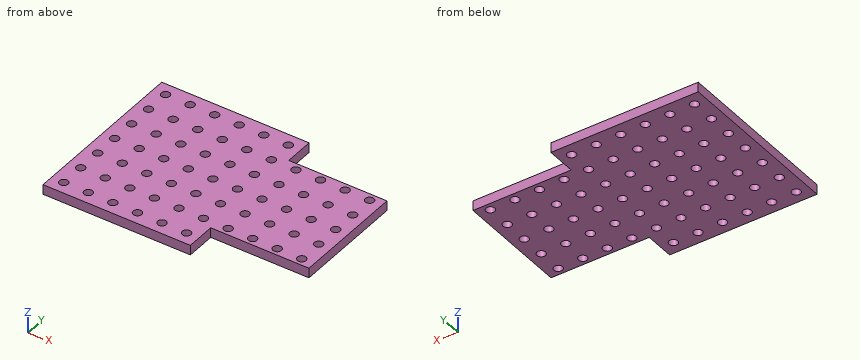
from build123d import *

# Parameters (mm, degrees)
ESQUISSE1_R        = 1.75
BOSS_EXTRU_1_DEPTH = 4


with BuildPart() as part:
    # Esquisse1 → Boss.-Extru.1 (new body)
    with BuildSketch(Plane.XY):
        Polygon((0, 0), (0, 70), (60, 70), (60, 58), (100, 58), (100, 12), (60, 12), (60, 0), align=None)
        with Locations((5, 5)):
            Circle(ESQUISSE1_R, mode=Mode.SUBTRACT)
        with Locations((15, 5)):
            Circle(ESQUISSE1_R, mode=Mode.SUBTRACT)
        with Locations((25, 5)):
            Circle(ESQUISSE1_R, mode=Mode.SUBTRACT)
        with Locations((35, 5)):
            Circle(ESQUISSE1_R, mode=Mode.SUBTRACT)
        with Locations((45, 5)):
            Circle(ESQUISSE1_R, mode=Mode.SUBTRACT)
        with Locations((55, 5)):
            Circle(ESQUISSE1_R, mode=Mode.SUBTRACT)
        with Locations((15, 15)):
            Circle(ESQUISSE1_R, mode=Mode.SUBTRACT)
        with Locations((25, 15)):
            Circle(ESQUISSE1_R, mode=Mode.SUBTRACT)
        with Locations((35, 15)):
            Circle(ESQUISSE1_R, mode=Mode.SUBTRACT)
        with Locations((45, 15)):
            Circle(ESQUISSE1_R, mode=Mode.SUBTRACT)
        with Locations((55, 15)):
            Circle(ESQUISSE1_R, mode=Mode.SUBTRACT)
        with Locations((65, 15)):
            Circle(ESQUISSE1_R, mode=Mode.SUBTRACT)
        with Locations((75, 15)):
            Circle(ESQUISSE1_R, mode=Mode.SUBTRACT)
        with Locations((85, 15)):
            Circle(ESQUISSE1_R, mode=Mode.SUBTRACT)
        with Locations((95, 15)):
            Circle(ESQUISSE1_R, mode=Mode.SUBTRACT)
        with Locations((15, 25)):
            Circle(ESQUISSE1_R, mode=Mode.SUBTRACT)
        with Locations((25, 25)):
            Circle(ESQUISSE1_R, mode=Mode.SUBTRACT)
        with Locations((35, 25)):
            Circle(ESQUISSE1_R, mode=Mode.SUBTRACT)
        with Locations((45, 25)):
            Circle(ESQUISSE1_R, mode=Mode.SUBTRACT)
        with Locations((55, 25)):
            Circle(ESQUISSE1_R, mode=Mode.SUBTRACT)
        with Locations((65, 25)):
            Circle(ESQUISSE1_R, mode=Mode.SUBTRACT)
        with Locations((75, 25)):
            Circle(ESQUISSE1_R, mode=Mode.SUBTRACT)
        with Locations((85, 25)):
            Circle(ESQUISSE1_R, mode=Mode.SUBTRACT)
        with Locations((95, 25)):
            Circle(ESQUISSE1_R, mode=Mode.SUBTRACT)
        with Locations((15, 35)):
            Circle(ESQUISSE1_R, mode=Mode.SUBTRACT)
        with Locations((25, 35)):
            Circle(ESQUISSE1_R, mode=Mode.SUBTRACT)
        with Locations((35, 35)):
            Circle(ESQUISSE1_R, mode=Mode.SUBTRACT)
        with Locations((45, 35)):
            Circle(ESQUISSE1_R, mode=Mode.SUBTRACT)
        with Locations((55, 35)):
            Circle(ESQUISSE1_R, mode=Mode.SUBTRACT)
        with Locations((65, 35)):
            Circle(ESQUISSE1_R, mode=Mode.SUBTRACT)
        with Locations((75, 35)):
            Circle(ESQUISSE1_R, mode=Mode.SUBTRACT)
        with Locations((85, 35)):
            Circle(ESQUISSE1_R, mode=Mode.SUBTRACT)
        with Locations((95, 35)):
            Circle(ESQUISSE1_R, mode=Mode.SUBTRACT)
        with Locations((15, 45)):
            Circle(ESQUISSE1_R, mode=Mode.SUBTRACT)
        with Locations((25, 45)):
            Circle(ESQUISSE1_R, mode=Mode.SUBTRACT)
        with Locations((35, 45)):
            Circle(ESQUISSE1_R, mode=Mode.SUBTRACT)
        with Locations((45, 45)):
            Circle(ESQUISSE1_R, mode=Mode.SUBTRACT)
        with Locations((55, 45)):
            Circle(ESQUISSE1_R, mode=Mode.SUBTRACT)
        with Locations((65, 45)):
            Circle(ESQUISSE1_R, mode=Mode.SUBTRACT)
        with Locations((75, 45)):
            Circle(ESQUISSE1_R, mode=Mode.SUBTRACT)
        with Locations((85, 45)):
            Circle(ESQUISSE1_R, mode=Mode.SUBTRACT)
        with Locations((95, 45)):
            Circle(ESQUISSE1_R, mode=Mode.SUBTRACT)
        with Locations((15, 55)):
            Circle(ESQUISSE1_R, mode=Mode.SUBTRACT)
        with Locations((25, 55)):
            Circle(ESQUISSE1_R, mode=Mode.SUBTRACT)
        with Locations((35, 55)):
            Circle(ESQUISSE1_R, mode=Mode.SUBTRACT)
        with Locations((45, 55)):
            Circle(ESQUISSE1_R, mode=Mode.SUBTRACT)
        with Locations((55, 55)):
            Circle(ESQUISSE1_R, mode=Mode.SUBTRACT)
        with Locations((65, 55)):
            Circle(ESQUISSE1_R, mode=Mode.SUBTRACT)
        with Locations((75, 55)):
            Circle(ESQUISSE1_R, mode=Mode.SUBTRACT)
        with Locations((85, 55)):
            Circle(ESQUISSE1_R, mode=Mode.SUBTRACT)
        with Locations((95, 55)):
            Circle(ESQUISSE1_R, mode=Mode.SUBTRACT)
        with Locations((15, 65)):
            Circle(ESQUISSE1_R, mode=Mode.SUBTRACT)
        with Locations((25, 65)):
            Circle(ESQUISSE1_R, mode=Mode.SUBTRACT)
        with Locations((35, 65)):
            Circle(ESQUISSE1_R, mode=Mode.SUBTRACT)
        with Locations((45, 65)):
            Circle(ESQUISSE1_R, mode=Mode.SUBTRACT)
        with Locations((55, 65)):
            Circle(ESQUISSE1_R, mode=Mode.SUBTRACT)
        with Locations((5, 15)):
            Circle(ESQUISSE1_R, mode=Mode.SUBTRACT)
        with Locations((5, 25)):
            Circle(ESQUISSE1_R, mode=Mode.SUBTRACT)
        with Locations((5, 35)):
            Circle(ESQUISSE1_R, mode=Mode.SUBTRACT)
        with Locations((5, 45)):
            Circle(ESQUISSE1_R, mode=Mode.SUBTRACT)
        with Locations((5, 55)):
            Circle(ESQUISSE1_R, mode=Mode.SUBTRACT)
        with Locations((5, 65)):
            Circle(ESQUISSE1_R, mode=Mode.SUBTRACT)
    extrude(amount=BOSS_EXTRU_1_DEPTH)


solid = part.part
Verification items for the finished model (mm, model axes). Round coordinates to 2 decimals unless told otherwise and drop trailing zeros. Write each loop counter-clockwise with the first axis right and the second up, starting at its lowest first coordinate (ties: lowest second). Pieces come first, ordered by that corner, then holes.
(1) Material ranges on line 1 (X direction, y = 61.5, z = 2); line 2 (Y direction, x = 91, z = 1.3), recorded low to high.
Returned:
line 1: x = 0 to 60
line 2: y = 12 to 58
(2) Section check B-B (x = 65). Enter the section's corners in (y, z).
Returned:
outline: (12, 0) - (13.25, 0) - (13.25, 4) - (12, 4) - close; (16.75, 0) - (23.25, 0) - (23.25, 4) - (16.75, 4) - close; (26.75, 0) - (33.25, 0) - (33.25, 4) - (26.75, 4) - close; (36.75, 0) - (43.25, 0) - (43.25, 4) - (36.75, 4) - close; (46.75, 0) - (53.25, 0) - (53.25, 4) - (46.75, 4) - close; (56.75, 0) - (58, 0) - (58, 4) - (56.75, 4) - close
(3) Depth check by flat-ended pin: pin 1 Ø1.5 at (x, z) = (61.5, 3) entering from +Y. Enter the tip coordinate at first touch or a pass-through.
Returned:
pin 1: stops at y = 58
(4) Section check A-A (x = 5). Give the number of separate pieces and of enclosed holes in the cut face, plus the area to 3 significant figures.
Returned:
separate pieces: 8
enclosed holes: 0
area: 182 mm2
